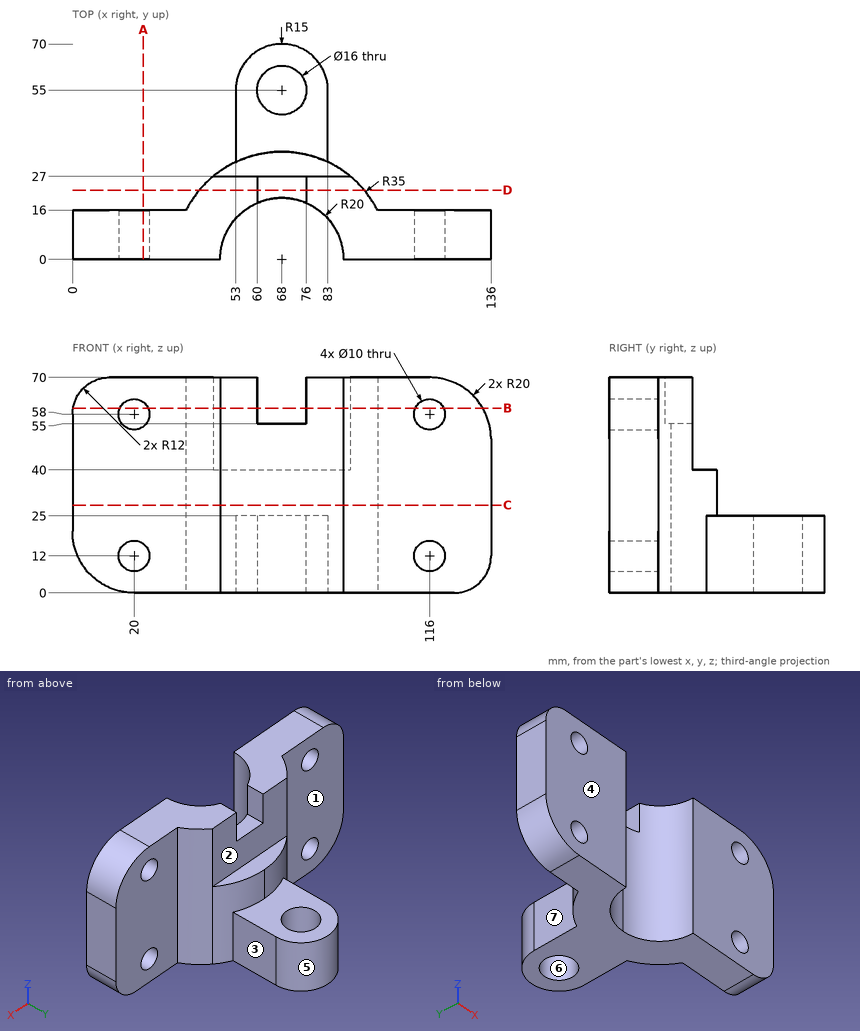
Check sheet for the drawn part. Datum: minimum x, y, z corner. Units: mm. A direction names the side the tool comes from. Round coordinates to 2 decimals unless told otherwise and drop trailing zeros. Order: outer loops, then holes, each group sorted by start corner. A loop starts at its lowest first (then second) coordinate and runs counter-clockwise, first axis right, second up.
1) Scan lines: line 1 (Z direction, x = 20, y = 10.5); line 2 (Y direction, x = 130, z = 34); line 3 (Z direction, x = 119, y = 13). Record each from-to range of solid material in increasing order.
2) Mould release check, pull along Y, two halves, no side actions. Record for the marked faces 4, 5, 6 and 7: +Y half, -Y half, draft (parallel to the pull), parting line (faces both ways), or undercut.
3) Section check A-A (x = 23). Record the boundary of the cut face in (y, z).
4) Section check B-B (z = 60). Record the boundary of the cut face in (x, y).
5) Section check D-D (y = 22.5). Record the boundary of the cut face in (x, z).
6) Tool access check on the marked faces 1, 2 and 3. Record the directions out of +Z, -Z, +X, -X, +Y, -Y that give a thin tool (end or side, any length) a straight path to the whole face; none if there is none.
7) Section check C-C (z = 28.5). Record the boundary of the cut face in (x, y).
8) Go/stop test with flat-tipped pins: pin 1 Ø7 at (x, y) = (65, 22.5) entering from +Z; pin 2 Ø2 at (x, z) = (73, 39) entering from -Y; pin 3 Ø11.5 at (x, z) = (20, 12) entering from +Y. Record where each tip stops, or that it passes through.
Result:
1. line 1: z = 0 to 7, 17 to 53, 63 to 70
1. line 2: y = 0 to 16
1. line 3: z = 0 to 8, 16 to 54, 62 to 69.77
2. face 4: -Y half
2. face 5: +Y half
2. face 6: undercut
2. face 7: draft
3. outline: (0, 0) - (16, 0) - (16, 8) - (0, 8) - close; (0, 16) - (16, 16) - (16, 54) - (0, 54) - close; (0, 62) - (16, 62) - (16, 70) - (0, 70) - close
4. outline: (0.17, 0) - (15.42, 0) - (15.42, 16) - (0.17, 16) - close; (24.58, 0) - (48, 0) arc R20 cw to (60, 18.33) - (60, 27) - (45.73, 27) arc R35 ccw to (36.87, 16) - (24.58, 16) - close; (76, 18.33) arc R20 cw to (88, 0) - (111.42, 0) - (111.42, 16) - (99.13, 16) arc R35 ccw to (90.27, 27) - (76, 27) - close; (120.58, 0) - (133.32, 0) - (133.32, 16) - (120.58, 16) - close
5. outline: (41.19, 0) - (94.81, 0) - (94.81, 70) - (76, 70) - (76, 55) - (60, 55) - (60, 70) - (41.19, 70) - close
6. face 1: +Z, -Z, -X, +Y
6. face 2: +Z, +X, -X, +Y
6. face 3: +Z, -Z, +X, +Y
7. outline: (0, 0) - (48, 0) arc R20 cw to (88, 0) - (136, 0) - (136, 16) - (99.13, 16) arc R35 ccw to (36.87, 16) - (0, 16) - close
8. pin 1: stops at z = 55
8. pin 2: stops at y = 19.08
8. pin 3: stops at y = 16
